```python
from build123d import *

# Parameters (mm, degrees)
T_LE_DE_BASE_PLI_E1_DEPTH = 1.5
CONG_1_R                  = 5
ESQUISSE2_W               = 103
ESQUISSE2_H               = 14
PATTE1_DEPTH              = 1.5
ESQUISSE5_R               = 1.5
ESQUISSE5_RX              = 9
ESQUISSE5_RY              = 8.5
ESQUISSE5_RX_2            = 6
ESQUISSE5_RY_2            = 4
ESQUISSE5_W               = 10
ESQUISSE5_H               = 4
ESQUISSE5_W_2             = 4
ESQUISSE5_H_2             = 1.2
ENL_V_MAT_EXTRU_1_DEPTH   = 1.5
ENL_V_MAT_EXTRU_3_DEPTH   = 169.577133681
CONG_2_R                  = 1
CONG_3_R                  = 2
ESQUISSE6_R               = 1.25
ESQUISSE6_R_2             = 1.5
ENL_V_MAT_EXTRU_2_DEPTH   = 1.5
CONG_5_R                  = 0.5
ESQUISSE11_R              = 1.6
ESQUISSE11_RX             = 54.51081151
ESQUISSE11_RY             = 20
ENL_V_MAT_EXTRU_4_DEPTH   = 169.004757327
CONG_4_R                  = 2


# Sheet-metal steps are written as plain solids
with BuildPart() as part:
    # Esquisse1 → Tôle de base pliée1 (new body)
    with BuildSketch(Plane(origin=(0, 0, 0), x_dir=(1, 0, 0), z_dir=(0, 1, 0))):
        with BuildLine():
            Line((0, 55), (-134, 55))
            Line((-134, 55), (-134, 38))
            Line((-134, 38), (-153.801820535, 38))
            ThreePointArc((-153.801820535, 38), (-147.637295096, 26.754721957), (-140.652052953, 16))
            Line((-140.652052953, 16), (0, 16))
            Line((0, 16), (0, 55))
        make_face()
    extrude(amount=-T_LE_DE_BASE_PLI_E1_DEPTH)

    # Congé1
    cong_1_edges = [part.edges().sort_by_distance(p)[0] for p in [
        (-134, -0.75, -38),
    ]]
    fillet(cong_1_edges, radius=CONG_1_R)

    # Esquisse2 → Patte1 (add)
    with BuildSketch(Plane(origin=(0, 0, 0), x_dir=(1, 0, 0), z_dir=(0, 1, 0))):
        with Locations((-51.5, 62)):
            Rectangle(ESQUISSE2_W, ESQUISSE2_H)
    extrude(amount=-PATTE1_DEPTH)

    # Esquisse5 → Enlèv. mat.-Extru.1 (cut)
    with BuildSketch(Plane(origin=(0, 0, 0), x_dir=(1, 0, 0), z_dir=(0, 1, 0))):
        with Locations(Location((-125, 45, 0), (0, 0, 270))):
            Circle(ESQUISSE5_R)
        with Locations(Location((-115, 45, 0), (0, 0, 90))):
            Circle(ESQUISSE5_R)
        with Locations(Location((-77.3, 54.5), (0, 0, 90))):
            Ellipse(ESQUISSE5_RX, ESQUISSE5_RY)
        with Locations(Location((-35, 52), (0, 0, -90))):
            Ellipse(ESQUISSE5_RX_2, ESQUISSE5_RY_2)
        with Locations((-98, 67)):
            Rectangle(ESQUISSE5_W, ESQUISSE5_H)
        with Locations((-132, 54.4)):
            Rectangle(ESQUISSE5_W_2, ESQUISSE5_H_2)
    extrude(amount=-ENL_V_MAT_EXTRU_1_DEPTH, mode=Mode.SUBTRACT)

    # Esquisse7 → Enlèv. mat.-Extru.3 (cut, through all)
    with BuildSketch(Plane.XZ.offset(1.5)):
        with BuildLine():
            Line((-94, -26.776862841), (-94, -34.127707598))
            Line((-94, -34.127707598), (-89.445593183, -44.717925725))
            Line((-89.445593183, -44.717925725), (-81.281078387, -40.954617932))
            ThreePointArc((-81.281078387, -40.954617932), (-76.561125557, -40.050559309), (-71.964476608, -41.452734458))
            Line((-71.964476608, -41.452734458), (-64.210600306, -46.087357996))
            Line((-64.210600306, -46.087357996), (-59, -36.743965137))
            Line((-59, -36.743965137), (-59, -27.99850523))
            Line((-59, -27.99850523), (-69.035694847, -22))
            Line((-69.035694847, -22), (-83.636572532, -22))
            Line((-83.636572532, -22), (-94, -26.776862841))
        make_face()
    extrude(amount=-ENL_V_MAT_EXTRU_3_DEPTH, mode=Mode.SUBTRACT)

    # Congé2
    cong_2_edges = [part.edges().sort_by_distance(p)[0] for p in [
        (-153.801820535, -0.75, -38),
        (-64.210600306, -0.75, -46.087357996),
        (-89.445593183, -0.75, -44.717925725),
        (-130, -0.75, -55),
    ]]
    fillet(cong_2_edges, radius=CONG_2_R)

    # Congé3
    cong_3_edges = [part.edges().sort_by_distance(p)[0] for p in [
        (-134, -0.75, -53.8),
        (-93, -0.75, -69),
        (-93, -0.75, -65),
        (-103, -0.75, -65),
        (-103, -0.75, -55),
        (-140.652052953, -0.75, -16),
        (-59, -0.75, -36.743965137),
        (-59, -0.75, -27.99850523),
        (-69.035694847, -0.75, -22),
        (-83.636572532, -0.75, -22),
        (-94, -0.75, -26.776862841),
        (-94, -0.75, -34.127707598),
    ]]
    fillet(cong_3_edges, radius=CONG_3_R - 0.0001)  # a hair under: the kernel refuses the full size

    # Esquisse6 → Enlèv. mat.-Extru.2 (cut)
    with BuildSketch(Plane(origin=(0, 0, 0), x_dir=(1, 0, 0), z_dir=(0, 1, 0))):
        with Locations(Location((-120.25, 37, 0), (0, 0, 270))):
            Circle(ESQUISSE6_R)
        with Locations(Location((-104.75, 37, 0), (0, 0, 270))):
            Circle(ESQUISSE6_R)
        with Locations(Location((-45.25, 37, 0), (0, 0, 270))):
            Circle(ESQUISSE6_R)
        with Locations(Location((-29.75, 37, 0), (0, 0, 270))):
            Circle(ESQUISSE6_R)
        with Locations(Location((-90, 55.15, 0), (0, 0, 270))):
            Circle(ESQUISSE6_R_2)
        with Locations(Location((-65, 55.15, 0), (0, 0, 270))):
            Circle(ESQUISSE6_R_2)
        with BuildLine():
            Line((-119, 24), (-106, 24))
            ThreePointArc((-106, 24), (-101.5, 19.5), (-106, 15))
            Line((-106, 15), (-119, 15))
            ThreePointArc((-119, 15), (-123.5, 19.5), (-119, 24))
        make_face()
        with BuildLine():
            Line((-44, 24), (-31, 24))
            ThreePointArc((-31, 24), (-26.5, 19.5), (-31, 15))
            Line((-31, 15), (-44, 15))
            ThreePointArc((-44, 15), (-48.5, 19.5), (-44, 24))
        make_face()
    extrude(amount=-ENL_V_MAT_EXTRU_2_DEPTH, mode=Mode.SUBTRACT)

    # Congé5
    cong_5_edges = [part.edges().sort_by_distance(p)[0] for p in [
        (-28.171572875, -0.75, -16),
        (-46.828427125, -0.75, -16),
        (-103.171572875, -0.75, -16),
        (-121.828427125, -0.75, -16),
    ]]
    fillet(cong_5_edges, radius=CONG_5_R)

    # Symétrie1: part across face


with BuildPart() as part_1:
    add(part.part)
    add(part.part.mirror(Plane(origin=(0, -0.75, -42.5), x_dir=(0, 0, 1), z_dir=(1, 0, 0))))

    # Esquisse11 → Enlèv. mat.-Extru.4 (cut, through all)
    with BuildSketch(Plane(origin=(0, 0, 0), x_dir=(1, 0, 0), z_dir=(0, 1, 0))):
        with Locations(Location((-8, 51, 0), (0, 0, 270))):
            Circle(ESQUISSE11_R)
        with Locations(Location((8, 51, 0), (0, 0, 270))):
            Circle(ESQUISSE11_R)
        with Locations(Location((-129, 20, 0), (0, 0, 270))):
            Circle(ESQUISSE11_R)
        with Locations(Location((-21, 20, 0), (0, 0, 270))):
            Circle(ESQUISSE11_R)
        with Locations(Location((21, 20, 0), (0, 0, 270))):
            Circle(ESQUISSE11_R)
        with Locations(Location((129, 20, 0), (0, 0, 270))):
            Circle(ESQUISSE11_R)
        with Locations(Location((-96, 20, 0), (0, 0, 270))):
            Circle(ESQUISSE11_R)
        with Locations(Location((-54, 20, 0), (0, 0, 270))):
            Circle(ESQUISSE11_R)
        with Locations(Location((54, 20, 0), (0, 0, 270))):
            Circle(ESQUISSE11_R)
        with Locations(Location((96, 20, 0), (0, 0, 270))):
            Circle(ESQUISSE11_R)
        with Locations((0, 75)):
            Ellipse(ESQUISSE11_RX, ESQUISSE11_RY)
    extrude(amount=-ENL_V_MAT_EXTRU_4_DEPTH, mode=Mode.SUBTRACT)

    # Congé4
    cong_4_edges = [part_1.edges().sort_by_distance(p)[0] for p in [
        (52, -0.75, -69),
        (-52, -0.75, -69),
    ]]
    fillet(cong_4_edges, radius=CONG_4_R)


solid = part_1.part
```
Model file for the job. Use its own axes, mm. A direction names the side the tool comes from. Give positions to 0.01 mm unless a question says otherwise; leave off trailing zeros.
1) Mould opens along Z. For faces 1 (the flat face through (64.208, -0.76, -24.886)), 2 (the flat face through (2, 0, -37)), 3 (the cylindrical face through (-147.57, -0.74, -26.64)), 4 (the cylindrical face through (-135, -1, -40)) say: +Z half, -Z half, draft (parallel to the pull), parting line (faces both ways), or undercut.
2) Saw through at A-A, the plane y = -1.15. Count the separate pieces of the cut face and the enclosed holes in it, then the cut area to 3 significant figures.
3) 3-axis set-ups, long thin cutter, end or side, ignore diameter. For faces 5 (the cylindrical face through (147.57, -0.74, -26.64)), 6 (the flat face through (-64.208, -0.76, -24.886)): which of +Z, -Z, +X, -X, +Y, -Y reach the whole face in a straight line?
4) Wall check: probe 1 along Z at (x, y) = (-129, -0.85); probe 2 along X at (y, z) = (-0.9, -43); probe 3 along X at (y, z) = (-0.65, -62.5). Give the ranges that are in metal, low to high.
5) Pin check, flat tips, straight feed: pin 1 (0.8 mm diameter, centred on x = 109.5, y = -0.5, fed in from +Z); pin 2 (2.5 mm diameter, centred on x = 125, z = -45, fed in from -Y). Stop position of each tip, or through.
Computed:
1. face 1: undercut
1. face 2: draft
1. face 3: +Z half
1. face 4: -Z half
2. separate pieces: 1
2. enclosed holes: 32
2. area: 10,000 mm2
3. face 5: +Z, +X, +Y, -Y
3. face 6: +Y, -Y
4. probe 1: z = -55 to -21.6, -18.4 to -16
4. probe 2: x = -134 to -90.18, -85.72 to -69.38, -62.49 to 62.49, 69.38 to 85.72, 90.18 to 134
4. probe 3: x = -103 to -81.19, -73.41 to -42.55, 42.55 to 73.41, 81.19 to 103
5. pin 1: stops at z = -24
5. pin 2: passes through
